```python
from build123d import *

# Parameters (mm, degrees)
SKETCH_1_R          = 27.5
EXTRUDE_1_DEPTH     = 3
SKETCH_1_3_R        = 25.4
EXTRUDE_2_DEPTH     = 7.1
SKETCH_1_4_R        = 22
EXTRUDE_3_DEPTH     = 10
SKETCH_1_5_R        = 13
CUT_EXTRUDE_1_DEPTH = 10


with BuildPart() as part:
    # 草图1 → 凸台-拉伸1 (new body)
    with BuildSketch(Plane.XY):
        Circle(SKETCH_1_R)
    extrude(amount=EXTRUDE_1_DEPTH)

    # 草图1<3> → 凸台-拉伸2 (add)
    with BuildSketch(Plane.XY):
        Circle(SKETCH_1_3_R)
    extrude(amount=EXTRUDE_2_DEPTH)

    # 草图1<4> → 凸台-拉伸3 (add)
    with BuildSketch(Plane.XY):
        Circle(SKETCH_1_4_R)
    extrude(amount=EXTRUDE_3_DEPTH)

    # 草图1<5> → 切除-拉伸1 (cut)
    with BuildSketch(Plane.XY):
        Circle(SKETCH_1_5_R)
    extrude(amount=CUT_EXTRUDE_1_DEPTH, mode=Mode.SUBTRACT)


solid = part.part
```
The listing builds one solid part. Answer for the finished solid, in the listing's coordinates (mm). A direction names the side the tool comes from. Coordinates: 2 decimals unless noted, no trailing zeros. Loops run counter-clockwise (first coordinate to the right, second up) from the corner with the lowest first, then second, coordinate; pieces in that order, holes last. Notation, with made-up numbers: (0.5, -14.75) - (36.5, -14.75) arc R23 ccw to (36.5, 2.25) - close; hole circle Ø1 at (88.5, 71). An arc over 180 degrees is marked (long way). Use a Markdown table: item, result. Add a question column.
1) The part is cut by section C-C, the plane z = 5.5. Give the vertices of the cut face in (x, y).
2) For faces 1 (the cylindrical face through (-4.769, -21.477, 8.53)), 2 (the cylindrical face through (-5.961, -26.846, 1.479)), determine the directions among +Z, -Z, +X, -X, +Y, -Y from which every point of the face is accessible in a straight line to the end or side of a thin tool.
3) The part is cut by section D-D, the plane x = 16. Give the vertices of the cut face in (y, z).
4) Find the intervals of material crossed by line 1 (Y direction, x = 0, z = 3.75); line 2 (Z direction, x = 18, y = 18.5); line 3 (Z direction, x = -11, y = 21), in increasing order.
5) The part is cut by section A-A, the plane y = 0. Give the vertices of the cut face in (x, z), and give its area (3 significant figures).
6) Given pin 1 (1.5 mm diameter, centred on x = 20, y = 22, fed in from -Z); pin 2 (4 mm diameter, centred on x = 5.5, z = 2.5, fed in from -Y); pin 3 (5 mm diameter, centred on y = 22, z = 7, fed in from -X); pin 4 (2 mm diameter, centred on x = 2, z = 4.5, fed in from +Y), each flat-ended and moving along its own axis, determine where each tip first touches the part or whether it passes through.
Here are the results:
| question | item | result |
|---|---|---|
| 1 | outline | circle Ø50.8 at (0, 0); hole circle Ø26 at (0, 0) |
| 2 | face 1 | +Z |
| 2 | face 2 | +Z, -Z |
| 3 | outline | (-22.37, 0) - (22.37, 0) - (22.37, 3) - (19.73, 3) - (19.73, 7.1) - (15.1, 7.1) - (15.1, 10) - (-15.1, 10) - (-15.1, 7.1) - (-19.73, 7.1) - (-19.73, 3) - (-22.37, 3) - close |
| 4 | line 1 | y = -25.4 to -13, 13 to 25.4 |
| 4 | line 2 | z = 0 to 3 |
| 4 | line 3 | z = 0 to 7.1 |
| 5 | outline | (-27.5, 0) - (-13, 0) - (-13, 10) - (-22, 10) - (-22, 7.1) - (-25.4, 7.1) - (-25.4, 3) - (-27.5, 3) - close; (13, 0) - (27.5, 0) - (27.5, 3) - (25.4, 3) - (25.4, 7.1) - (22, 7.1) - (22, 10) - (13, 10) - close |
| 5 | area | 241 mm^2 |
| 6 | pin 1 | passes through |
| 6 | pin 2 | stops at y = -27.28 |
| 6 | pin 3 | stops at x = -16.28 |
| 6 | pin 4 | stops at y = 25.38 |
